from build123d import *

# Parameters (mm, degrees)
BOSS_EXTRUDE2_DEPTH     = 4
CUT_EXTRUDE1_DEPTH      = 3
BOSS_EXTRUDE4_DEPTH     = 24
CUT_EXTRUDE3_DEPTH      = 25
CUT_EXTRUDE3_DEPTH_BACK = 183.067360447
SKETCH8_OUTSIDE_W       = 285.221
SKETCH8_OUTSIDE_H       = 85.963
CUT_EXTRUDE5_START      = -2
SKETCH15_R              = 6
CUT_EXTRUDE5_DEPTH      = 2
FILLET2_START           = -5
FILLET2_DEPTH           = 3
CUT_EXTRUDE4_DEPTH      = 2
FILLET1_R               = 1.5
FILLET1_OF_MIRROR2_R    = 1.5
CHAMFER2_SIZE           = 2
M4_CLEARANCE_HOLE1_D    = 4.5


with BuildPart() as part:
    # Sketch1 → Boss-Extrude2 (new, symmetric)
    with BuildSketch(Plane.XY):
        with BuildLine():
            Line((-174.954279742, 10), (0, 10))
            ThreePointArc((0, 10), (23.648322027, 11.894462409), (46.69345503, 17.529528282))
            ThreePointArc((46.69345503, 17.529528282), (54.142205969, 14.082195987), (51.181218931, 6.427096624))
            ThreePointArc((51.181218931, 6.427096624), (27.055536633, -3.305079876), (1.870729257, -9.823460289))
            ThreePointArc((1.870729257, -9.823460289), (0.711714534, -9.974640967), (-0.457023425, -9.98955102))
            Line((-0.457023425, -9.98955102), (-175.228493797, -1.993730612))
            ThreePointArc((-175.228493797, -1.993730612), (-180.95271219, 4.137142857), (-174.954279742, 10))
        make_face()
    extrude(amount=BOSS_EXTRUDE2_DEPTH, both=True)

    # Sketch4 → Cut-Extrude1 (cut)
    with BuildSketch(Plane.XY.offset(4)):
        with BuildLine():
            ThreePointArc((-174.954279742, 10), (-180.95271219, 4.137142857), (-175.228493797, -1.993730612))
            Line((-175.228493797, -1.993730612), (-122.27878396, -4.416187605))
            ThreePointArc((-122.27878396, -4.416187605), (-115.249733713, 2.05087413), (-109.954279742, 10))
            Line((-109.954279742, 10), (-174.954279742, 10))
        make_face()
    extrude(amount=-CUT_EXTRUDE1_DEPTH, mode=Mode.SUBTRACT)

    # Sweep2: sweep along a curve in space
    with BuildLine() as sweep2_path:
        ThreePointArc((-122.27878396, -4.416187605, 1), (-115.249733713, 2.05087413, 1), (-109.954279742, 10, 1))
    # Sketch9 → Sweep2 (sweep)
    with BuildSketch(Plane(origin=(-18.347220561, -36.300543819, 0), x_dir=(0.8924819376724606, -0.45108313083999296, 0), z_dir=(0.4510831308399929, 0.8924819376724605, 0))):
        Polygon((-102.643039948, -1), (-102.643039948, -4), (-111.643039948, -1), align=None)
    sweep(path=sweep2_path.line)

    # Sketch10 → Boss-Extrude4 (add)
    with BuildSketch(Plane(origin=(-82.616299838, -59.493723404, 0), x_dir=(0, 0, 1), z_dir=(-0.8114878209620178, -0.584369332212357, 0))):
        Polygon((1, 67.87228887), (4, 67.87228887), (1, 76.87228887), align=None)
    extrude(amount=BOSS_EXTRUDE4_DEPTH)

    # Sketch8 outside → Cut-Extrude3 (cut, two sides: drawn at the far end of the back side and taken through both)
    with BuildSketch(Plane.XY.offset(-4).offset(-CUT_EXTRUDE3_DEPTH_BACK)):
        with Locations((-63.1875, -0.3035)):
            Rectangle(SKETCH8_OUTSIDE_W, SKETCH8_OUTSIDE_H)
        with BuildLine():
            Line((0, 10), (-174.954279742, 10))
            ThreePointArc((-174.954279742, 10), (-180.95271219, 4.137142857), (-175.228493797, -1.993730612))
            Line((-175.228493797, -1.993730612), (-0.457023425, -9.98955102))
            ThreePointArc((-0.457023425, -9.98955102), (0.711714534, -9.974640967), (1.870729257, -9.823460289))
            ThreePointArc((1.870729257, -9.823460289), (27.055536633, -3.305079876), (51.181218931, 6.427096624))
            ThreePointArc((51.181218931, 6.427096624), (54.142205969, 14.082195987), (46.69345503, 17.529528282))
            ThreePointArc((46.69345503, 17.529528282), (23.648322027, 11.894462409), (0, 10))
        make_face(mode=Mode.SUBTRACT)
    extrude(amount=CUT_EXTRUDE3_DEPTH + CUT_EXTRUDE3_DEPTH_BACK, mode=Mode.SUBTRACT)

    # Sketch15 → Cut-Extrude5 (cut)
    with BuildSketch(Plane(origin=(0, 0, -4), x_dir=(-1, 0, 0), z_dir=(0, 0, -1)).offset(CUT_EXTRUDE5_START)):
        with Locations((-48.579466687, 11.83365609)):
            Circle(SKETCH15_R)
    extrude(amount=CUT_EXTRUDE5_DEPTH, mode=Mode.SUBTRACT)

    # Fillet2: read off the stored shape, not the designer's step
    # Fillet2 outline → Fillet2 (cut)
    with BuildSketch(Plane.XY.offset(FILLET2_START)):
        with BuildLine():
            ThreePointArc((40.241823664, 15.554681857), (42.163553049, 15.077161786), (42.732589809, 13.180515689))
            ThreePointArc((42.732589809, 13.180515689), (44.143492284, 15.873721819), (46.69345503, 17.529528282))
            ThreePointArc((46.69345503, 17.529528282), (43.478853193, 16.505470524), (40.241823664, 15.554681857))
        make_face()
        with BuildLine():
            ThreePointArc((45.110606605, 6.938044817), (45.943997016, 5.103233461), (44.757331788, 3.474461553))
            ThreePointArc((44.757331788, 3.474461553), (47.982323267, 4.922391468), (51.181218931, 6.427096624))
            ThreePointArc((51.181218931, 6.427096624), (48.076241077, 5.854796334), (45.110606605, 6.938044817))
        make_face()
    extrude(amount=FILLET2_DEPTH, mode=Mode.SUBTRACT)

    # Sketch14 → Cut-Extrude4 (cut)
    with BuildSketch(Plane.XY.offset(4)):
        with BuildLine():
            Line((-14.832396974, 6), (-39.944961285, 6))
            ThreePointArc((-39.944961285, 6), (-43.908510482, 0.633863605), (-48.921261535, -3.768121054))
            Line((-48.921261535, -3.768121054), (-15.091112688, -5.315855326))
            ThreePointArc((-15.091112688, -5.315855326), (-15.995819862, 0.365714286), (-14.832396974, 6))
        make_face()
        with BuildLine():
            ThreePointArc((-62.816908131, -3.132393183), (-54.164987884, -0.012926968), (-47.205713301, 6))
            Line((-47.205713301, 6), (-100.774922993, 6))
            ThreePointArc((-100.774922993, 6), (-102.783982304, 2.310087116), (-105.095731275, -1.198130822))
            Line((-105.095731275, -1.198130822), (-62.816908131, -3.132393183))
        make_face()
        with BuildLine():
            ThreePointArc((37.636421144, 10.71573201), (26.161853464, 8.260130678), (14.532481339, 6.693802069))
            ThreePointArc((14.532481339, 6.693802069), (15.849901808, 2.186461221), (15.802019276, -2.509220357))
            ThreePointArc((15.802019276, -2.509220357), (27.792022964, 1.161065661), (39.522801968, 5.590513918))
            ThreePointArc((39.522801968, 5.590513918), (38.25647934, 8.034191359), (37.636421144, 10.71573201))
        make_face()
    cut_extrude4 = extrude(amount=-CUT_EXTRUDE4_DEPTH, mode=Mode.SUBTRACT)

    # Fillet1
    fillet1_edges = [part.edges().sort_by_distance(p)[0] for p in [
        (14.532481339, 6.693802069, 3),
        (37.636421144, 10.71573201, 3),
        (39.522801968, 5.590513918, 3),
        (15.802019276, -2.509220357, 3),
        (-39.944961285, 6, 3),
        (-14.832396974, 6, 3),
        (-15.091112688, -5.315855326, 3),
        (-48.921261535, -3.768121054, 3),
        (-47.205713301, 6, 3),
        (-62.816908131, -3.132393183, 3),
        (-105.095731275, -1.198130822, 3),
        (-100.774922993, 6, 3),
    ]]
    fillet(fillet1_edges, radius=FILLET1_R)

    # Mirror2: Cut-Extrude4 across plane
    add(cut_extrude4.mirror(Plane.XY), mode=Mode.SUBTRACT)

    # Fillet1 of Mirror2
    fillet1_of_mirror2_edges = [part.edges().sort_by_distance(p)[0] for p in [
        (14.532481339, 6.693802069, -3),
        (37.636421144, 10.71573201, -3),
        (39.522801968, 5.590513918, -3),
        (15.802019276, -2.509220357, -3),
        (-39.944961285, 6, -3),
        (-14.832396974, 6, -3),
        (-15.091112688, -5.315855326, -3),
        (-48.921261535, -3.768121054, -3),
        (-47.205713301, 6, -3),
        (-62.816908131, -3.132393183, -3),
        (-105.095731275, -1.198130822, -3),
        (-100.774922993, 6, -3),
    ]]
    fillet(fillet1_of_mirror2_edges, radius=FILLET1_OF_MIRROR2_R)

    # Chamfer2
    # the kernel refuses this chamfer: 2 mm, written as the material it takes off along each edge
    with BuildSketch(Plane(origin=(-35.543855882, 186.645745489, -4), x_dir=(0.42492369608644903, -0.9052291712623004, 0), z_dir=(0.9052291712623004, 0.42492369608644903, 0))) as chamfer2_piece_1:
        Polygon((200 - CHAMFER2_SIZE, 0), (200, -CHAMFER2_SIZE), (200, 0), align=None)
    revolve(axis=Axis((-35.543855882, 186.645745489, -4), (0, 0, -1)), revolution_arc=14.36382118, mode=Mode.SUBTRACT)
    with BuildSketch(Plane(origin=(-0.457023425, -9.98955102, -4), x_dir=(0.04570234246318501, 0.9989551020408164, 0), z_dir=(-0.9989551020408164, 0.04570234246318502, 0)), Plane(origin=(-174.954279742, 10, -4), x_dir=(0, -1, 0), z_dir=(1, 0, 0))) as chamfer2_piece_2:
        Polygon((CHAMFER2_SIZE, 0), (0, -CHAMFER2_SIZE), (0, 0), align=None)
    extrude(amount=174.954279742, mode=Mode.SUBTRACT)
    with BuildSketch(Plane(origin=(0, 158.546658899, -4), x_dir=(0, -1, 0), z_dir=(-1, 0, 0))) as chamfer2_piece_3:
        Polygon((148.546658899 + CHAMFER2_SIZE, 0), (148.546658899, CHAMFER2_SIZE), (148.546658899, 0), align=None)
    revolve(axis=Axis((0, 158.546658899, -4), (0, 0, 1)), revolution_arc=17.7019097, mode=Mode.SUBTRACT)
    with BuildSketch(Plane(origin=(-174.954279742, 4, -4), x_dir=(-0.045702342463191735, -0.998955102040816, 0), z_dir=(0.998955102040816, -0.045702342463191735, 0))) as chamfer2_piece_4:
        Polygon((6 - CHAMFER2_SIZE, 0), (6, -CHAMFER2_SIZE), (6, 0), align=None)
    revolve(axis=Axis((-174.954279742, 4, -4), (0, 0, -1)), revolution_arc=177.380536242, mode=Mode.SUBTRACT)
    with BuildSketch(Plane(origin=(0, 0, -4), x_dir=(0.187072925695108, -0.9823460288879232, 0), z_dir=(0.9823460288879232, 0.187072925695108, 0))) as chamfer2_piece_5:
        Polygon((10 - CHAMFER2_SIZE, 0), (10, -CHAMFER2_SIZE), (10, 0), align=None)
    revolve(axis=Axis((0, 0, -4), (0, 0, -1)), revolution_arc=13.401476298, mode=Mode.SUBTRACT)

    # M4 Clearance Hole1 (through all)
    with Locations(Plane.XY.offset(4)):
        with Locations((0, 0), (48.579466687, 11.83365609), (-174.954279742, 4)):
            Hole(M4_CLEARANCE_HOLE1_D / 2)


solid = part.part
Build history of the part. All positions in model axes, mm. A direction names the side the tool comes from. Round coordinates to 2 decimals unless told otherwise and drop trailing zeros. Write each loop counter-clockwise with the first axis right and the second up, starting at its lowest first coordinate (ties: lowest second). Pieces come first, ordered by that corner, then holes. Notation, with made-up numbers: M -23,-28.5 L 21,-28.5 A27 ccw 21,-7.5 Z; hole C 41.5,72 d10. An arc over 180 degrees is marked long. Use CSV: the item, a comma, the result in double quotes.
1. Wall check: probe 1 along Y at (x, z) = (0, -1.75); probe 2 along Z at (x, y) = (-117, -3.5); probe 3 along Y at (x, z) = (2, -2.75). Give the ranges that are in metal, low to high. Write a range as from..to.
Reply:
probe 1,"y = -10..-2.25, 2.25..10"
probe 2,"z = -3.16..4"
probe 3,"y = -9.04..-1.03, 1.03..9.26"
2. Tool access for faces 1 (the face through (-151, 5, 1)), 2 (the face through (21.1, 10.7, -2.8)), 3 (the face through (27, 4, -2)), 4 (the face through (-77, 2, 2)), 5 (the face through (-69, 10, 1)): list every direction of +Z, -Z, +X, -X, +Y, -Y with a clear straight run to the whole face (end or side of a thin tool).
Reply:
face 1,"+Z, -X, +Y"
face 2,"-Z, -X, +Y"
face 3,"-Z"
face 4,"+Z"
face 5,"+Z, -Z, -X, +Y"
3. Saw through at A-A (z = -0.75). Give the cut face in (x, y), plus the area to 3 significant figures.
Reply:
outline,"M -175.23,-1.99 L -0.46,-9.99 A10 ccw 1.87,-9.82 A200 ccw 51.18,6.43 A6 ccw 46.69,17.53 A148.55 cw 0,10 L -174.95,10 A6 ccw Z; hole C -174.95,4 d4.5; hole C 0,0 d4.5; hole C 48.58,11.83 d4.5"
area,"3,660 mm²"
4. Saw through at B-B (x = -26.5). Give the cut face in (y, z).
Reply:
outline,"M -8.8,-2 L -6.8,-4 L -4.79,-4 L -4.79,-2 L 6,-2 L 6,-4 L 8,-4 L 10,-2 L 10,4 L 6,4 L 6,2 L -4.79,2 L -4.79,4 L -8.8,4 Z"
5. Flat gauge pins, fed straight in: pin 1 (0.6 mm diameter, centred on x = -28.5, z = -2.5, fed in from -Y); pin 2 (7 mm diameter, centred on x = 0, y = 0, fed in from -Z); pin 3 (11.5 mm diameter, centred on x = 50.5, y = 10, fed in from -Z); pin 4 (4.5 mm diameter, centred on x = -71.5, y = 1, fed in from +Z). Where does each tip first touch, or does it go through?
Reply:
pin 1,"stops at y = -8.51"
pin 2,"stops at z = -4"
pin 3,"stops at z = -2"
pin 4,"stops at z = 2"
